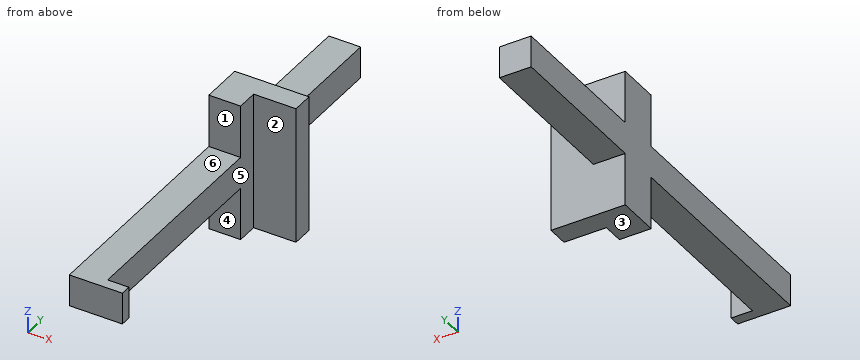
from build123d import *

# Parameters (mm, degrees)
BOSS_EXTRUDE1_DEPTH = 3
SKETCH2_W           = 3
SKETCH2_H           = 4
BOSS_EXTRUDE2_DEPTH = 5
SKETCH5_W           = 13
SKETCH5_H           = 2
BOSS_EXTRUDE4_DEPTH = 4


with BuildPart() as part:
    # Sketch1 → Boss-Extrude1 (new body)
    with BuildSketch(Plane.XY):
        Polygon((0, 0), (0, 40), (3, 40), (3, 1), (5, 1), (5, 0), align=None)
    extrude(amount=BOSS_EXTRUDE1_DEPTH)

    # Sketch2 → Boss-Extrude2 (add)
    with BuildSketch(Plane.XY.offset(3)):
        with Locations((1.5, 23.5)):
            Rectangle(SKETCH2_W, SKETCH2_H)
    boss_extrude2 = extrude(amount=BOSS_EXTRUDE2_DEPTH)

    # Mirror1: Boss-Extrude2 across plane
    add(boss_extrude2.mirror(Plane.XY.offset(1.5)))

    # Sketch5 → Boss-Extrude4 (add)
    with BuildSketch(Plane(origin=(3, 0, 0), x_dir=(0, 0, -1), z_dir=(1, 0, 0))):
        with Locations((-1.5, 24.5)):
            Rectangle(SKETCH5_W, SKETCH5_H)
    extrude(amount=BOSS_EXTRUDE4_DEPTH)


solid = part.part
Source: CAD feature listing. Evaluate the final solid. Frame: model axes, mm. Face numbers are marked on the shaded views. A direction names the side the tool comes from. Round coordinates to 2 decimals unless told otherwise and drop trailing zeros. Loops run counter-clockwise (first coordinate to the right, second up) from the corner with the lowest first, then second, coordinate; pieces in that order, holes last. Notation, with made-up numbers: M 51,-9 L 104,-9 A18 cw 104,21 Z; hole C -20.5,5.25 d10. An arc over 180 degrees is marked long. Return JSON: item names as keys, results as strings. Group by question number.
1. Mould query, pull axis Y, two halves, no side actions, for the marked faces 1, 2 and 3. Classes: released by +Y, released by -Y, zero draft, split by the parting line, or undercut.
2. Pin query (flat end, axial travel): pin 1 (2.5 mm diameter, centred on x = 2, y = 30.5, fed in from -Z); pin 2 (2 mm diameter, centred on x = 2.5, z = -2, fed in from +Y); pin 3 (2.5 mm diameter, centred on y = 30.5, z = 2, fed in from +X). Return the tip coordinate at first contact, or that it passes through.
3. Material intervals for line 1 along Z through (x, y) = (2.25, 6.5); line 2 along Y through (x, z) = (6.5, 1.25), sorted ascending. Write a range as from..to.
4. Section query C-C on z = -1. Output: boundary loops of the cut face in (x, y).
5. Reachability of the marked faces 4, 5 and 6 from +Z, -Z, +X, -X, +Y, -Y: full face, straight path, thin tool, end or side. Return the list, or none.
6. Section query B-B on x = 1. Output: boundary loops of the cut face in (y, z), and give its area (3 significant figures).
7. Section query D-D on y = 4. Output: boundary loops of the cut face in (x, z), and give its area (3 significant figures).
8. Section query A-A on x = 4.25. Output: boundary loops of the cut face in (y, z), and give its area (3 significant figures).
Checks:
{
 "1": {"face 1": "released by -Y", "face 2": "undercut", "face 3": "zero draft"},
 "2": {"pin 1": "stops at z = 0", "pin 2": "stops at y = 25.5", "pin 3": "stops at x = 3"},
 "3": {"line 1": "z = 0..3", "line 2": "y = 23.5..25.5"},
 "4": {"outline": "M 0,21.5 L 3,21.5 L 3,23.5 L 7,23.5 L 7,25.5 L 0,25.5 Z"},
 "5": {"face 4": "-Z, +X, -X, -Y", "face 5": "+Z, -Z, +X", "face 6": "+Z, +X, -X, -Y"},
 "6": {"outline": "M 0,0 L 21.5,0 L 21.5,-5 L 25.5,-5 L 25.5,0 L 40,0 L 40,3 L 25.5,3 L 25.5,8 L 21.5,8 L 21.5,3 L 0,3 Z", "area": "160 mm²"},
 "7": {"outline": "M 0,0 L 3,0 L 3,3 L 0,3 Z", "area": "9.00 mm²"},
 "8": {"outline": "M 0,0 L 1,0 L 1,3 L 0,3 Z; M 23.5,-5 L 25.5,-5 L 25.5,8 L 23.5,8 Z", "area": "29.0 mm²"}
}
